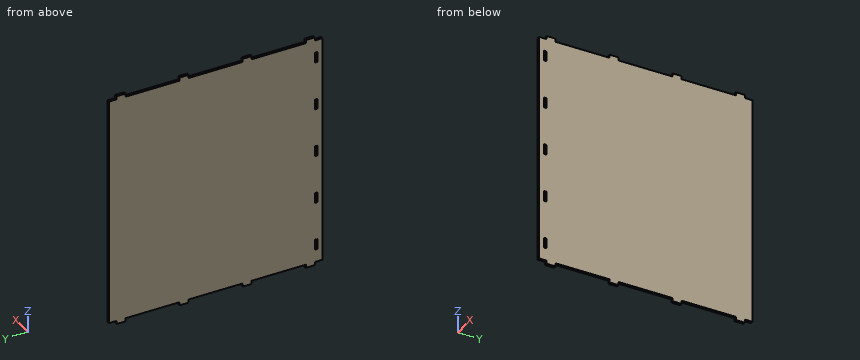
Autodesk Inventor part; units mm, degrees
ref_plane "YZ Plane" through (0, 0, 0) normal (1, 0, 0) x (0, 1, 0)
ref_plane "XZ Plane" through (0, 0, 0) normal (0, 1, 0) x (-1, 0, 0)
ref_plane "XY Plane" through (0, 0, 0) normal (0, 0, 1) x (1, 0, 0)
sketch "Sketch1" plane through (0, 0, 0) normal (1, 0, 0) x (0, 1, 0)
  line L0 (0, 0) -> (830, 0) construction
  line L1 (830, 0) -> (830, -900)
  line L2 (830, -900) -> (0, -900) construction
  line L3 (0, -900) -> (0, 0)
  line L4 (800, 0) -> (765, 0) construction
  line L5 (765, 0) -> (765, 12.6635)
  line L6 (765, 12.6635) -> (800, 12.6635)
  line L7 (800, 12.6635) -> (800, 0)
  line L8 (555, 0) -> (520, 0) construction
  line L9 (520, 0) -> (520, 12.6635)
  line L10 (520, 12.6635) -> (555, 12.6635)
  line L11 (555, 12.6635) -> (555, 0)
  line L12 (310, 0) -> (275, 0) construction
  line L13 (275, 0) -> (275, 12.6635)
  line L14 (275, 12.6635) -> (310, 12.6635)
  line L15 (310, 12.6635) -> (310, 0)
  line L16 (65, 0) -> (30, 0) construction
  line L17 (30, 0) -> (30, 12.6635)
  line L18 (30, 12.6635) -> (65, 12.6635)
  line L19 (65, 12.6635) -> (65, 0)
  line L20 (830, -450) -> (0, -450) construction
  line L21 (800, -900) -> (765, -900) construction
  line L22 (765, -900) -> (765, -912.6635)
  line L23 (765, -912.6635) -> (800, -912.6635)
  line L24 (800, -912.6635) -> (800, -900)
  line L25 (555, -900) -> (520, -900) construction
  line L26 (520, -900) -> (520, -912.6635)
  line L27 (520, -912.6635) -> (555, -912.6635)
  line L28 (555, -912.6635) -> (555, -900)
  line L29 (310, -900) -> (275, -900) construction
  line L30 (275, -900) -> (275, -912.6635)
  line L31 (275, -912.6635) -> (310, -912.6635)
  line L32 (310, -912.6635) -> (310, -900)
  line L33 (65, -900) -> (30, -900) construction
  line L34 (30, -900) -> (30, -912.6635)
  line L35 (30, -912.6635) -> (65, -912.6635)
  line L36 (65, -912.6635) -> (65, -900)
  line L37 (830, -900) -> (800, -900)
  line L38 (765, -900) -> (555, -900)
  line L39 (520, -900) -> (310, -900)
  line L40 (275, -900) -> (65, -900)
  line L41 (30, -900) -> (0, -900)
  line L42 (830, 0) -> (800, 0)
  line L43 (765, 0) -> (555, 0)
  line L44 (520, 0) -> (310, 0)
  line L45 (275, 0) -> (65, 0)
  line L46 (30, 0) -> (0, 0)
  line L47 (20, -50) -> (30, -50)
  line L48 (30, -50) -> (30, -90)
  line L49 (30, -90) -> (20, -90)
  line L50 (20, -90) -> (20, -50)
  line L51 (20, -240) -> (30, -240)
  line L52 (30, -240) -> (30, -280)
  line L53 (30, -280) -> (20, -280)
  line L54 (20, -280) -> (20, -240)
  line L55 (20, -430) -> (30, -430)
  line L56 (30, -430) -> (30, -470)
  line L57 (30, -470) -> (20, -470)
  line L58 (20, -470) -> (20, -430)
  line L59 (20, -620) -> (30, -620)
  line L60 (30, -620) -> (30, -660)
  line L61 (30, -660) -> (20, -660)
  line L62 (20, -660) -> (20, -620)
  line L63 (20, -810) -> (30, -810)
  line L64 (30, -810) -> (30, -850)
  line L65 (30, -850) -> (20, -850)
  line L66 (20, -850) -> (20, -810)
  dimension "d0" = 900
  dimension "d1" = 830
  dimension "d2" = 35
  dimension "d3" = 30
  dimension "d4" = 210
  dimension "d5" = 210
  dimension "d6" = 210
  dimension "d7" = 30
  dimension "d11" = 40
  dimension "d12" = 10
  dimension "d15" = 40
  dimension "d16" = 10
  dimension "d17" = 40
  dimension "d18" = 10
  dimension "d19" = 40
  dimension "d20" = 10
  dimension "d21" = 40
  dimension "d22" = 10
  dimension "d23" = 150
  dimension "d24" = 150
  dimension "d25" = 150
  dimension "d26" = 150
  dimension "d27" = 50
  dimension "d28" = 50
  dimension "d31" = 20
extrude "Extrusion3" add sketch "Sketch1" along normal blind 10
properties part number "Fundo" material "Wood (Oak)"
Could you check a few things on this model? Use its own coordinates, in mm. Coordinates: 2 decimals unless noted, no trailing zeros. Loops run counter-clockwise (first coordinate to the right, second up) from the corner with the lowest first, then second, coordinate; pieces in that order, holes last.
1) Imagine slicing it at B-B (y = 587.5). List the corners of the cut face in (x, z) for me.
Reported:
outline: (0, -900) - (10, -900) - (10, 0) - (0, 0) - close
2) Please list where these lines run through material, in increasing order: line 1 along Y through (x, z) = (5, -445); line 2 along Z through (x, y) = (1, 465.5).
Reported:
line 1: y = 0 to 20, 30 to 830
line 2: z = -900 to 0
3) Imagine slicing it at A-A (x = 3.25). State how many separate pieces and enclosed holes the cut face has, and give its area (3 significant figures).
Reported:
separate pieces: 1
enclosed holes: 5
area: 749,000 mm2
4) Will these pins go through, and if not, where does the flat tip stop? pin 1 Ø5 at (x, y) = (6, 24.5) entering from +Z; pin 2 Ø5 at (x, z) = (6, 6.5) entering from -Y.
Reported:
pin 1: stops at z = 0
pin 2: stops at y = 30
